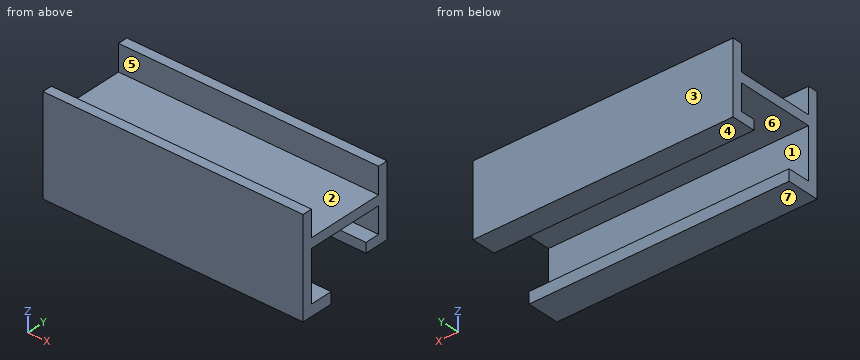
from build123d import *

# Parameters (mm, degrees)
EXTRUDE_1_DEPTH = 80


with BuildPart() as part:
    # Эскиз1 → Бобышка-Вытянуть1 (new, symmetric)
    with BuildSketch(Plane(origin=(0, 0, 0), x_dir=(0, 0, -1), z_dir=(1, 0, 0))):
        Polygon((-30, -24), (-30, -30), (30, -30), (30, -10), (23, -10), (23, -24), (8, -24), (-8, -24), (-8, 24), (8, 24), (8, 15), (14, 15), (14, 30), (-30, 30), (-30, 24), (-14, 24), (-14, -24), align=None)
    extrude(amount=EXTRUDE_1_DEPTH, both=True)


solid = part.part
Read the model definition and answer for the solid it produces. Units are mm, in the model's axes. Face numbers are marked on the shaded views. A direction names the side the tool comes from. Give positions to 0.01 mm unless a question says otherwise; leave off trailing zeros. Loops run counter-clockwise (first coordinate to the right, second up) from the corner with the lowest first, then second, coordinate; pieces in that order, holes last. Notation, with made-up numbers: (50, 65.5) - (54, 65.5) arc R19 ccw to (54, 73.5) - close; hole circle Ø10 at (1.5, 73.25). An arc over 180 degrees is marked (long way). Answer as CSV lines item,"result". Start each with the question number.
1) Determine the mould class of the marked faces 1, 2, 3 and 4 for opening direction Y: released by +Y, released by -Y, zero draft, split by the parting line, or undercut.
2) Find section D-D (y = -7.5). Write down the section's boundary in (x, z), then the cut area to 3 significant figures.
3) Each of these flat-tipped pins is pushed along its axis until it touches: pin 1 Ø8 at (x, y) = (25, 6) entering from -Z; pin 2 Ø5.5 at (x, z) = (16, -26) entering from +Y; pin 3 Ø7.5 at (x, y) = (-14.5, 25) entering from -Z. Where does it stop, or does it pass through?
4) Straight lines are drawn through the part: L1, parallel to Y at x = -31, z = 6.5; L2, parallel to Z at x = -70.5, y = -18.5; L3, parallel to Y at x = 59, z = -11.5. For each, find the intervals that lie inside material, in ascending order. Write a range as from..to.
5) Which of the six approach directions +Z, -Z, +X, -X, +Y, -Y give full straight-line access (tool end or side, diameter ignored) to the marked faces 5, 6 and 7?
6) Find section A-A (y = 21). Write down the section's boundary in (x, z).
7) Find section B-B (z = -5). Write down the section's boundary in (x, y), then the cut area to 3 significant figures.
8) Find section C-C (x = -7.5). Write down the section's boundary in (y, z).
Findings below:
1,face 1,"undercut"
1,face 2,"undercut"
1,face 3,"released by +Y"
1,face 4,"zero draft"
2,outline,"(-80, 8) - (80, 8) - (80, 14) - (-80, 14) - close"
2,area,"960 mm^2"
3,pin 1,"z = 8"
3,pin 2,"y = -10"
3,pin 3,"z = -14"
4,L1,"-30..-24, 24..30"
4,L2,"-30..-23, 8..14"
4,L3,"-30..-24, 15..30"
5,face 5,"+Z, +X, -X"
5,face 6,"+X, -X"
5,face 7,"-Z, +X, -X, +Y, -Y"
6,outline,"(-80, -14) - (80, -14) - (80, -8) - (-80, -8) - close; (-80, 8) - (80, 8) - (80, 14) - (-80, 14) - close"
7,outline,"(-80, -30) - (80, -30) - (80, -24) - (-80, -24) - close; (-80, 24) - (80, 24) - (80, 30) - (-80, 30) - close"
7,area,"1,920 mm^2"
8,outline,"(-30, -30) - (-10, -30) - (-10, -23) - (-24, -23) - (-24, 8) - (24, 8) - (24, -8) - (15, -8) - (15, -14) - (30, -14) - (30, 30) - (24, 30) - (24, 14) - (-24, 14) - (-24, 30) - (-30, 30) - close"
